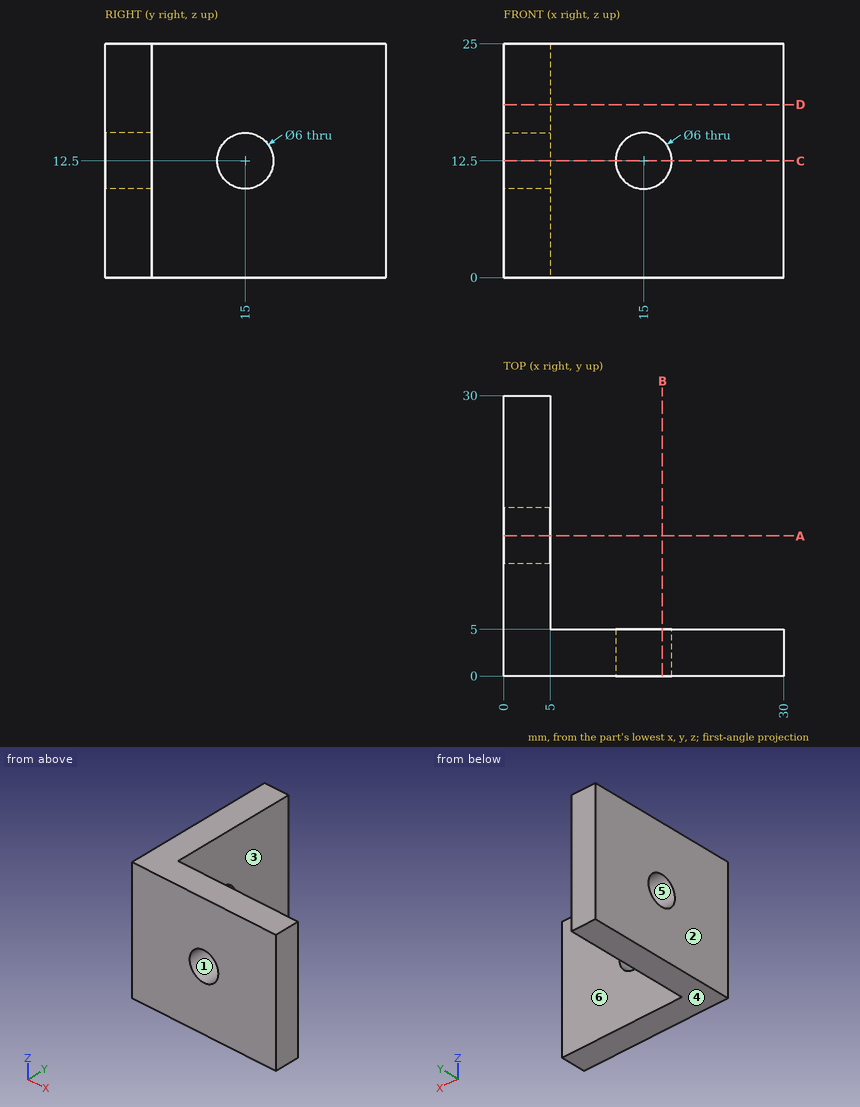
Source: three-view drawing plus pictorial views. Frame: mm from the lowest corner of the part. A direction names the side the tool comes from. Coordinates: 2 decimals unless noted, no trailing zeros. Write each loop counter-clockwise with the first axis right and the second up, starting at its lowest first coordinate (ties: lowest second). Pieces come first, ordered by that corner, then holes. Notation, with made-up numbers: (67.5, 81.25) - (85.5, 81.25) arc R18 ccw to (85.5, 99.25) - close; hole circle Ø10 at (16.25, 64). An arc over 180 degrees is marked (long way). Answer as a JSON object with one key per item and string values.
Q1. Section query C-C, the plane z = 12.5. Output: boundary loops of the cut face in (x, y).
Ans:
{"outline": "(0, 0) - (12, 0) - (12, 5) - (5, 5) - (5, 12) - (0, 12) - close; (0, 18) - (5, 18) - (5, 30) - (0, 30) - close; (18, 0) - (30, 0) - (30, 5) - (18, 5) - close"}
Q2. Section query D-D, the plane z = 18.5. Output: boundary loops of the cut face in (x, y), plus the area to 3 significant figures.
Ans:
{"outline": "(0, 0) - (30, 0) - (30, 5) - (5, 5) - (5, 30) - (0, 30) - close", "area": "275 mm2"}
Q3. Material intervals for line 1 (Z direction, x = 15, y = 3.8); line 2 (Y direction, x = 2.4, z = 12.5); line 3 (Y direction, x = 21, z = 3), sorted ascending. Write a range as [from, to].
Ans:
{"line 1": "z = [0, 9.5], [15.5, 25]", "line 2": "y = [0, 12], [18, 30]", "line 3": "y = [0, 5]"}
Q4. First-contact query: pin 1 Ø8 at (y, z) = (15, 12.5) entering from -X; pin 2 Ø12 at (x, z) = (23.5, 21) entering from +Y. Flat tips, straight axial feed; report the tip coordinate or a pass-through.
Ans:
{"pin 1": "stops at x = 0", "pin 2": "stops at y = 5"}
Q5. Set-up query: the marked faces 5 and 6. Return all of +Z, -Z, +X, -X, +Y, -Y with unobstructed straight access to the full face (end or side cutting, diameter ignored); none if empty.
Ans:
{"face 5": "+X, -X", "face 6": "+Z, -Z, +X, +Y"}
Q6. Section query A-A, the plane y = 15. Output: boundary loops of the cut face in (x, z).
Ans:
{"outline": "(0, 0) - (5, 0) - (5, 9.5) - (0, 9.5) - close; (0, 15.5) - (5, 15.5) - (5, 25) - (0, 25) - close"}
Q7. Draft query along X for the marked faces 1, 2, 3 and 4. Return one class per face: released by +X, released by -X, zero draft, split by the parting line, or undercut.
Ans:
{"face 1": "undercut", "face 2": "released by -X", "face 3": "released by +X", "face 4": "zero draft"}
Q8. Section query B-B, the plane x = 17. Output: boundary loops of the cut face in (y, z).
Ans:
{"outline": "(0, 0) - (5, 0) - (5, 10.26) - (0, 10.26) - close; (0, 14.74) - (5, 14.74) - (5, 25) - (0, 25) - close"}
